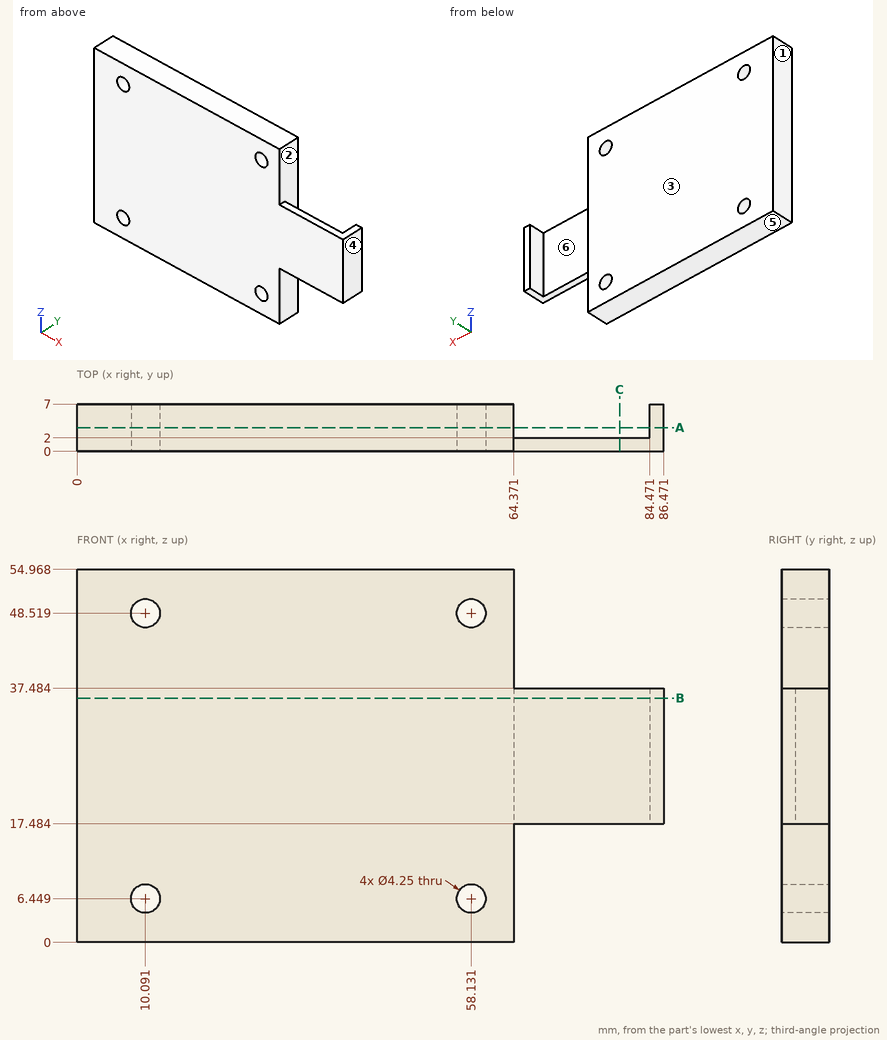
Geometry check sheet. Reference: drawing and pictorial views, mm from the part's lowest x, y, z. A direction names the side the tool comes from. Coordinates: 2 decimals unless noted, no trailing zeros. Order: outer loops, then holes, each group sorted by start corner. A loop starts at its lowest first (then second) coordinate and runs counter-clockwise, first axis right, second up.
Item 1: Section check C-C (x = 80). Enter the section's corners in (y, z).
Item 2: Section check B-B (z = 36). Enter the section's corners in (x, y), plus the area to 3 significant figures.
Item 3: Scan lines: line 1 along X through (y, z) = (4.5, 31); line 2 along Z through (x, y) = (60, 6.25) (1 decimal); line 3 along Z through (x, y) = (11, 2). Record each from-to range of solid material in increasing order.
Item 4: Tool access check on the marked faces 5 and 6. Record the directions out of +Z, -Z, +X, -X, +Y, -Y that give a thin tool (end or side, any length) a straight path to the whole face; none if there is none.
Item 5: Section check A-A (y = 3.5). Count the separate pieces of the cut face and the enclosed holes in it, plus the area to 3 significant figures.
Item 6: Mould release check, pull along X, two halves, no side actions. Record for the marked faces 1, 2, 3 and 4: released by +X, released by -X, zero draft, split by the parting line, or undercut.
Item 7: Depth check by flat-ended pin: pin 1 (5 mm diameter, centred on x = 10.09, z = 48.52, fed in from -Y); pin 2 (3.5 mm diameter, centred on x = 10.09, z = 6.45, fed in from +Y); pin 3 (4 mm diameter, centred on y = 3, z = 12, fed in from +X). Enter the tip coordinate at first touch or a pass-through.
Check sheet entries:
1. outline: (0, 17.48) - (2, 17.48) - (2, 37.48) - (0, 37.48) - close
2. outline: (0, 0) - (86.47, 0) - (86.47, 7) - (84.47, 7) - (84.47, 2) - (64.37, 2) - (64.37, 7) - (0, 7) - close
2. area: 505 mm2
3. line 1: x = 0 to 64.37, 84.47 to 86.47
3. line 2: z = 0 to 5.4, 7.5 to 47.5, 49.5 to 55
3. line 3: z = 0 to 4.53, 8.37 to 46.6, 50.44 to 54.97
4. face 5: -Z, +X, -X, +Y, -Y
4. face 6: +Z, -Z, +Y
5. separate pieces: 2
5. enclosed holes: 4
5. area: 3,520 mm2
6. face 1: released by -X
6. face 2: undercut
6. face 3: zero draft
6. face 4: released by +X
7. pin 1: stops at y = 0
7. pin 2: passes through
7. pin 3: stops at x = 64.37
